from build123d import *

# Parameters (mm, degrees)
F1_DEPTH = 152.4
F3_R     = 1.27
F4_DEPTH = 3.81
F6_DEPTH = 3.81
F7_R     = 1.27
F8_R     = 1.27


with BuildPart() as f1:
    # F0 (on Front) → F1 (new body, symmetric)
    with BuildSketch(Plane.XZ):
        Polygon((0, 50.8), (0, 0), (50.8, 0), (50.8, 3.175), (3.175, 3.175), (3.175, 50.8), align=None)
    extrude(amount=F1_DEPTH, both=True)

    # F3
    f3_edges = [f1.edges().sort_by_distance(p)[0] for p in [
        (3.175, 0, 50.8),
        (1.5875, 152.4, 50.8),
        (0, 0, 50.8),
        (1.5875, -152.4, 50.8),
    ]]
    fillet(f3_edges, radius=F3_R)

    # F2 (on face) → F4 (cut)
    with BuildSketch(Plane.XY.offset(3.175)):
        Polygon((50.8, 152.4), (3.175, 152.4), (50.8, 104.775), align=None)
    extrude(amount=-F4_DEPTH, mode=Mode.SUBTRACT)

    # F5 (on face) → F6 (cut)
    with BuildSketch(Plane.XY.offset(3.175)):
        Polygon((50.8, -104.775), (3.175, -152.4), (50.8, -152.4), align=None)
    extrude(amount=-F6_DEPTH, mode=Mode.SUBTRACT)

    # F7
    f7_edges = [f1.edges().sort_by_distance(p)[0] for p in [
        (50.8, -104.775, 1.5875),
        (50.8, 0, 3.175),
        (50.8, 104.775, 1.5875),
        (50.8, 0, 0),
    ]]
    fillet(f7_edges, radius=F7_R)

    # F8
    f8_edges = [f1.edges().sort_by_distance(p)[0] for p in [
        (0, 0, 0),
    ]]
    fillet(f8_edges, radius=F8_R)


solid = f1.part
Read the model definition and answer for the solid it produces. Units are mm, in the model's axes. A direction names the side the tool comes from. Round coordinates to 2 decimals unless told otherwise and drop trailing zeros. Loops run counter-clockwise (first coordinate to the right, second up) from the corner with the lowest first, then second, coordinate; pieces in that order, holes last. Notation, with made-up numbers: (76, -1.5) - (107, -1.5) arc R11 ccw to (107, 14.5) - close; hole circle Ø10 at (65.5, 66). An arc over 180 degrees is marked (long way). One line per question, with ' | ' between items. Start each with the question number.
Q1. Find the intervals of material crossed by L1, parallel to X at y = -63, z = 34 (3 decimals), in increasing order.
Q2. Flat-ended cylindrical pins translate along their axes: pin 1 (1 mm diameter, centred on y = 28.5, z = 24.5, fed in from +X) (3 decimals); pin 2 (5 mm diameter, centred on x = 12, y = -81.5, fed in from +Z) (3 decimals). Find the tip coordinate at first contact, or state that the pin passes through.
Q3. For faces 1 (the flat face through (25, -2, 0)), 2 (the flat face through (3.175, -2, 26)), determine the directions among +Z, -Z, +X, -X, +Y, -Y from which every point of the face is accessible in a straight line to the end or side of a thin tool.
Q4. Section C-C on x = 26 is taken. Give the vertices of the cut face in (y, z) (3 decimals), plus the area to 3 significant figures.
Q5. Section A-A on y = 91 is taken. Give the vertices of the cut face in (x, z) (3 decimals).
Q6. Section B-B on z = 7.5 is taken. Give the vertices of the cut face in (x, y) (3 decimals), plus the area to 3 significant figures.
Q7. Section D-D on y = -113.5 is taken. Give the vertices of the cut face in (x, z) (3 decimals), plus the area to 3 significant figures.
Established:
1) L1: 0 to 3.175
2) pin 1: x = 3.175 | pin 2: z = 3.175
3) face 1: -Z, +X, -X, +Y, -Y | face 2: +Z, +X, +Y, -Y
4) outline: (-129.575, 0) - (129.575, 0) - (129.575, 3.175) - (-129.575, 3.175) - close | area: 823 mm²
5) outline: (0, 1.27) arc R1.27 ccw to (1.27, 0) - (49.53, 0) arc R1.27 ccw to (50.8, 1.27) - (50.8, 1.905) arc R1.27 ccw to (49.53, 3.175) - (3.175, 3.175) - (3.175, 49.53) arc R1.27 ccw to (1.905, 50.8) - (1.27, 50.8) arc R1.27 ccw to (0, 49.53) - close
6) outline: (0, -152.4) - (3.175, -152.4) - (3.175, 152.4) - (0, 152.4) - close | area: 968 mm²
7) outline: (0, 1.27) arc R1.27 ccw to (1.27, 0) - (42.075, 0) - (42.075, 3.175) - (3.175, 3.175) - (3.175, 49.53) arc R1.27 ccw to (1.905, 50.8) - (1.27, 50.8) arc R1.27 ccw to (0, 49.53) - close | area: 284 mm²
